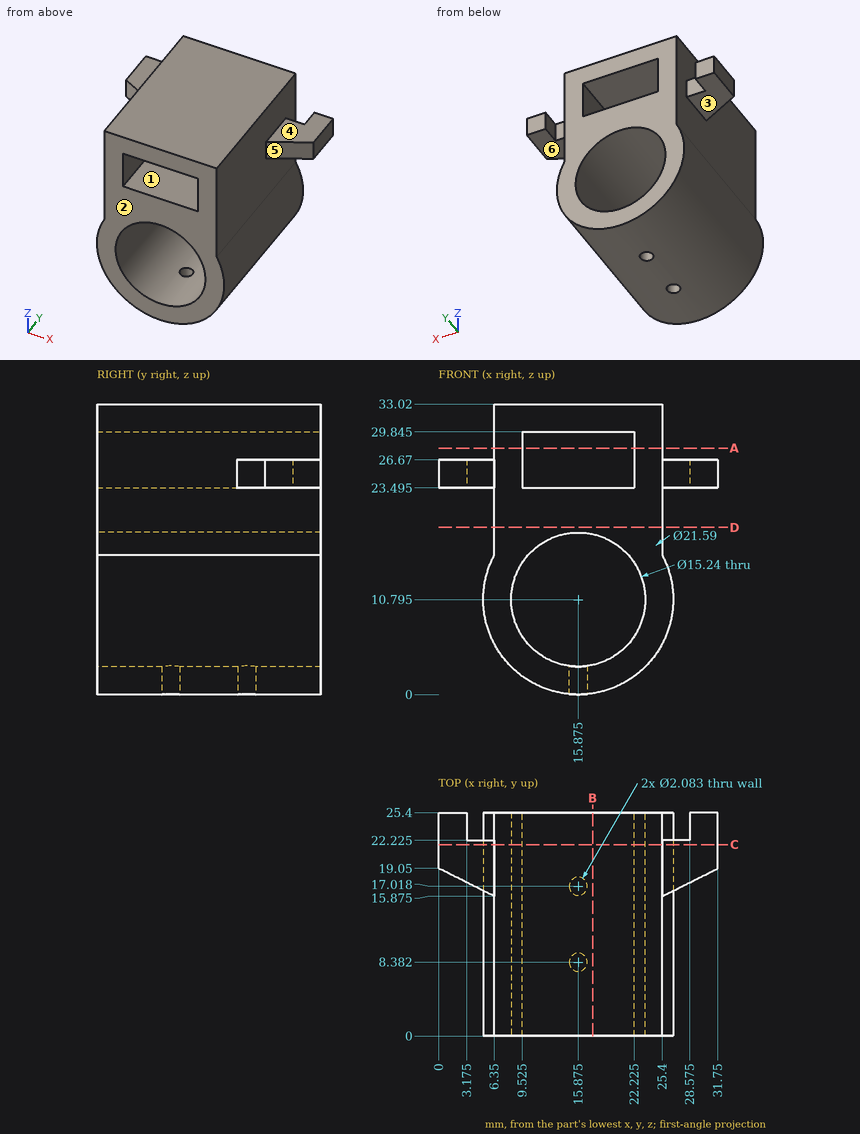
Check sheet for the drawn part. Datum: minimum x, y, z corner. Units: mm. A direction names the side the tool comes from. Round coordinates to 2 decimals unless told otherwise and drop trailing zeros. Loops run counter-clockwise (first coordinate to the right, second up) from the corner with the lowest first, then second, coordinate; pieces in that order, holes last. Notation, with made-up numbers: (55, 66.25) - (85, 66.25) arc R31 ccw to (85, 103.25) - close; hole circle Ø6 at (86.25, 85). An arc over 180 degrees is marked (long way). Write each question's results on one line, items separated by ' | '. Start each with the question number.
Q1. Access from +Z, -Z, +X, -X, +Y, -Y to the whole of each face (thin tool, end or side, straight path). Record for the marked faces 1, 2 and 3.
Q2. Cross-section at C-C on y = 21.75. Enter the section's corners in (x, z) (3 decimals), and give its area (3 significant figures).
Q3. Cross-section at A-A on z = 28. Enter the section's corners in (x, y) (3 decimals).
Q4. Release check for a two-part mould opening along Z. For the marked faces 4, 5 and 6 record: +Z half, -Z half, draft (parallel to the pull), parting line (faces both ways), or undercut.
Q5. Cross-section at D-D on z = 19. Enter the section's corners in (x, y).
Q6. Gauge pin test, flat ends, axial feed: P1, Ø1.9, axis at y = 17.5, z = 27, coming from the -X side; P2, Ø2, axis at x = 9, y = 8.5, coming from the -Z side; P3, Ø2, axis at x = 11.5, z = 6.5, coming from the -Y side; P4, Ø5, axis at y = 16, z = 24, coming from the +X side. Record the tip position at first contact, or that the pin passes through.
Q7. Thickness scan on line 1 (Z direction, x = 21, y = 7.75) (1 decimal); line 2 (Z direction, x = 14, y = 21.25) (1 decimal); line 3 (X direction, y = 15.25, z = 28) (3 decimals). Record the ranges inside material, lowest first. Write a range as [from, to].
Q8. Cross-section at B-B on x = 17.5. State how many separate pieces and enclosed holes the cut face has, and give its area (3 significant figures).
Answers below:
1) face 1: +Y, -Y | face 2: +Z, -Z, +X, -X, -Y | face 3: -X, +Y, -Y
2) outline: (0, 23.495) - (6.35, 23.495) - (6.35, 15.875) arc R10.795 ccw (long way) to (25.4, 15.875) - (25.4, 23.495) - (31.75, 23.495) - (31.75, 26.67) - (25.4, 26.67) - (25.4, 33.02) - (6.35, 33.02) - (6.35, 26.67) - (0, 26.67) - close; hole circle Ø15.24 at (15.875, 10.795); hole (9.525, 23.495) - (22.225, 23.495) - (22.225, 29.845) - (9.525, 29.845) - close | area: 392 mm²
3) outline: (6.35, 0) - (9.525, 0) - (9.525, 25.4) - (6.35, 25.4) - close; (22.225, 0) - (25.4, 0) - (25.4, 25.4) - (22.225, 25.4) - close
4) face 4: +Z half | face 5: draft | face 6: undercut
5) outline: (6.35, 0) - (25.4, 0) - (25.4, 25.4) - (6.35, 25.4) - close
6) P1: stops at x = 1.32 | P2: stops at z = 1.74 | P3: passes through | P4: stops at x = 30.65
7) line 1: z = [1.3, 5.2], [16.4, 23.5], [29.8, 33] | line 2: z = [0.2, 3.4], [18.2, 23.5], [29.8, 33] | line 3: x = [6.35, 9.525], [22.225, 25.4]
8) separate pieces: 3 | enclosed holes: 0 | area: 296 mm²
